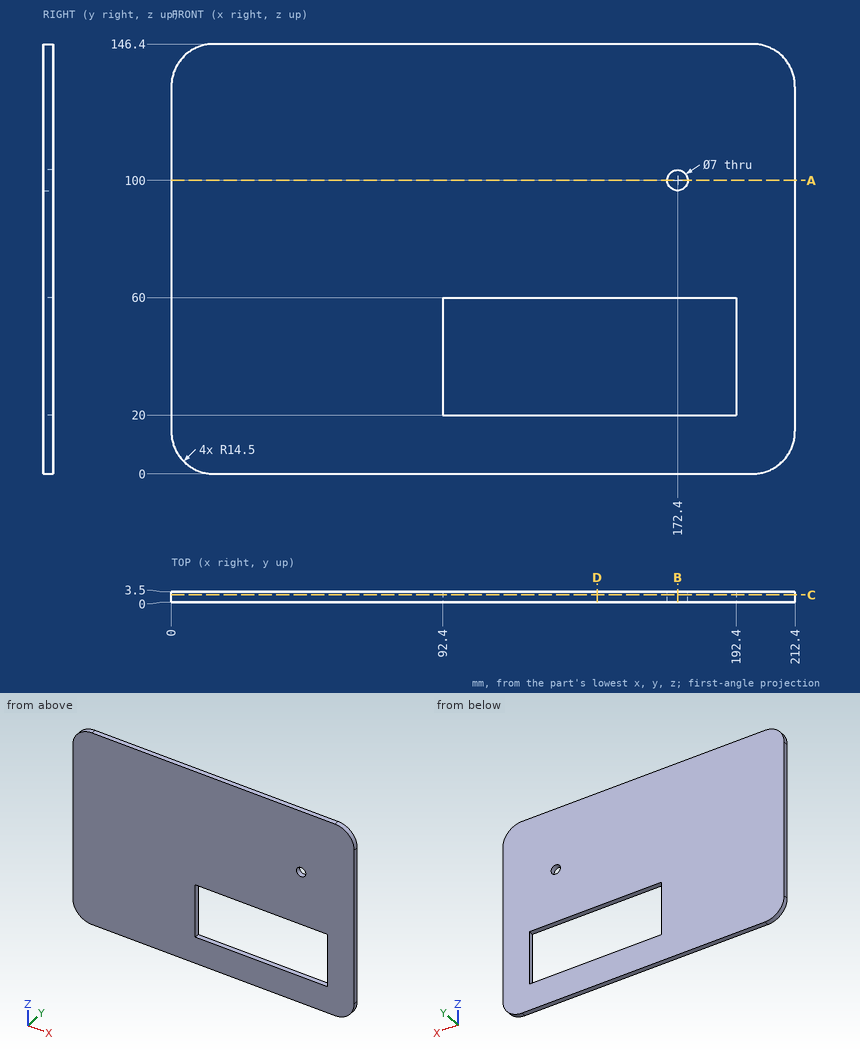
The figure shows three views and two pictorial views of one solid part (mm, origin at its lowest corner). Answer the questions. Round coordinates to 2 decimals unless told otherwise and drop trailing zeros. Loops run counter-clockwise (first coordinate to the right, second up) from the corner with the lowest first, then second, coordinate; pieces in that order, holes last. Notation, with made-up numbers: (37.25, 49) - (57.25, 49) arc R6 cw to (57.25, 58) - close; hole circle Ø1 at (-17, 18). An arc over 180 degrees is marked (long way). One line per question, with ' | ' between items. Start each with the question number.
Q1. Section B-B on x = 172.4 is taken. Give the vertices of the cut face in (y, z), plus the area to 3 significant figures.
Q2. Find the intervals of material crossed by L1, parallel to X at y = 1.7, z = 100; L2, parallel to Z at x = 95.5, y = 0.5; L3, parallel to Z at x = 173.5, y = 2.45, in increasing order.
Q3. Section C-C on y = 2.45 is taken. Give the vertices of the cut face in (x, z).
Q4. Section A-A on z = 100 is taken. Give the vertices of the cut face in (x, y), plus the area to 3 significant figures.
Q5. Section D-D on x = 145 is taken. Give the vertices of the cut face in (y, z).
Established:
1) outline: (0, 0) - (3.5, 0) - (3.5, 20) - (0, 20) - close; (0, 60) - (3.5, 60) - (3.5, 96.5) - (0, 96.5) - close; (0, 103.5) - (3.5, 103.5) - (3.5, 146.4) - (0, 146.4) - close | area: 348 mm²
2) L1: 0 to 168.9, 175.9 to 212.4 | L2: 0 to 20, 60 to 146.4 | L3: 0 to 20, 60 to 96.68, 103.32 to 146.4
3) outline: (0, 14.5) arc R14.5 ccw to (14.5, 0) - (197.9, 0) arc R14.5 ccw to (212.4, 14.5) - (212.4, 131.9) arc R14.5 ccw to (197.9, 146.4) - (14.5, 146.4) arc R14.5 ccw to (0, 131.9) - close; hole (92.4, 20) - (192.4, 20) - (192.4, 60) - (92.4, 60) - close; hole circle Ø7 at (172.4, 100)
4) outline: (0, 0) - (168.9, 0) - (168.9, 3.5) - (0, 3.5) - close; (175.9, 0) - (212.4, 0) - (212.4, 3.5) - (175.9, 3.5) - close | area: 719 mm²
5) outline: (0, 0) - (3.5, 0) - (3.5, 20) - (0, 20) - close; (0, 60) - (3.5, 60) - (3.5, 146.4) - (0, 146.4) - close
